from build123d import *

# Parameters (mm, degrees)
F0_W     = 22.5
F0_H     = 13
F1_DEPTH = 20
F2_R     = 7.75
F3_DEPTH = 12
F4_R     = 2


with BuildPart() as f1:
    # F0 (on Top) → F1 (new body)
    with BuildSketch(Plane.XY):
        with Locations((11.25, 6.5)):
            Rectangle(F0_W, F0_H)
    extrude(amount=F1_DEPTH)

    # F2 (on face) → F3 (cut)
    with BuildSketch(Plane.XZ):
        with Locations((11.25, 10)):
            Circle(F2_R)
    extrude(amount=-F3_DEPTH, mode=Mode.SUBTRACT)

    # F4
    f4_edges = [f1.edges().sort_by_distance(p)[0] for p in [
        (22.5, 6.5, 20),
        (22.5, 6.5, 0),
        (0, 6.5, 20),
        (0, 6.5, 0),
    ]]
    fillet(f4_edges, radius=F4_R)


solid = f1.part
Design review of the part built by this model. Coordinates are the model's own, in mm. Give positions to 0.01 mm unless a question says otherwise; leave off trailing zeros. Write each loop counter-clockwise with the first axis right and the second up, starting at its lowest first coordinate (ties: lowest second). Pieces come first, ordered by that corner, then holes. Notation, with made-up numbers: M -21.5,40.25 L 6.5,40.25 A21 cw 6.5,46.25 Z; hole C 43,64 d1. An arc over 180 degrees is marked long. Return JSON: item names as keys, results as strings. Group by question number.
Item 1: Wall thickness on line 1 along Z through (x, y) = (11.25, 7.5); line 2 along Y through (x, z) = (9.75, 4.25); line 3 along X through (y, z) = (6.75, 4.5): over which ranges is each line inside the solid? List them lowest first.
Item 2: Take a section at C-C (z = 10). Give the boundary of the cut face in (x, y), plus the area to 4 significant figures.
Item 3: Clearance check with a flat-ended pin moving along its axis: pin 1 Ø12 at (x, z) = (10, 9.5) entering from -Y. State where the tip first meets the part, or that it passes through.
Item 4: Take a section at A-A (y = 8). Give the boundary of the cut face in (x, z).
Item 5: Take a section at B-B (x = 11.25). Give the boundary of the cut face in (y, z), plus the area to 3 significant figures.
Item 6: The part is to be moulded in two halves that separate along Z. For faces 1 (the flat face through (0, 6, 10)), 2 (the cylindrical face through (5.54, 5.92, 15.24)), 3 (the flat face through (11, 7, 20)), 4 (the flat face through (11, 12, 10)), say which applies: pulls with the +Z half, pulls with the -Z half, needs draft (parallel to the pull), parting line crosses it, or undercut.
Return value:
{
 "1": {"line 1": "z = 0 to 2.25, 17.75 to 20", "line 2": "y = 12 to 13", "line 3": "x = 0 to 5.79, 16.71 to 22.5"},
 "2": {"outline": "M 0,0 L 3.5,0 L 3.5,12 L 19,12 L 19,0 L 22.5,0 L 22.5,13 L 0,13 Z", "area": "106.5 mm2"},
 "3": {"pin 1": "stops at y = 12"},
 "4": {"outline": "M 0,2 A2 ccw 2,0 L 20.5,0 A2 ccw 22.5,2 L 22.5,18 A2 ccw 20.5,20 L 2,20 A2 ccw 0,18 Z; hole C 11.25,10 d15.5"},
 "5": {"outline": "M 0,0 L 13,0 L 13,20 L 0,20 L 0,17.75 L 12,17.75 L 12,2.25 L 0,2.25 Z", "area": "74.0 mm2"},
 "6": {"face 1": "needs draft", "face 2": "undercut", "face 3": "pulls with the +Z half", "face 4": "undercut"}
}
